Autodesk Fusion 360 part; units mm, degrees
box "BoxPrimitive1" add length 35 width 12 height 12 placed x (0, 0, -1) y (-1, 0, 0) z (0, 1, 0) at (12, 0, 0)
box "BoxPrimitive2" add length 12 width 35 height 12 placed x (0, 0, -1) y (-1, 0, 0) z (0, 1, 0) at (35, 0, 0)
box "BoxPrimitive3" add length 12 width 12 height 35 placed x (0, 0, -1) y (-1, 0, 0) z (0, 1, 0) at (12, 0, 0)
cylinder "CylinderPrimitive1" cut diameter 3 height 15 placed x (1, 0, 0) y (0, 0, -1) z (0, 1, 0) at (30, 0, -5)
cylinder "CylinderPrimitive2" cut diameter 3 height 15 placed x (1, 0, 0) y (0, 0, -1) z (0, 1, 0) at (20, 0, -5)
cylinder "CylinderPrimitive3" cut diameter 3 height 15 placed x (1, 0, 0) y (0, 0, -1) z (0, 1, 0) at (5, 0, -30)
cylinder "CylinderPrimitive4" cut diameter 3 height 15 placed x (1, 0, 0) y (0, 0, -1) z (0, 1, 0) at (5, 0, -20)
cylinder "CylinderPrimitive5" cut diameter 3 height 15 placed x (0, 0, -1) y (0, 1, 0) z (1, 0, 0) at (0, 5, -30)
cylinder "CylinderPrimitive6" cut diameter 3 height 15 placed x (0, 0, -1) y (0, 1, 0) z (1, 0, 0) at (0, 5, -20)
cylinder "CylinderPrimitive7" cut diameter 3 height -15 placed x (0, 1, 0) y (1, 0, 0) z (0, 0, -1) at (30, 5, -12)
cylinder "CylinderPrimitive8" cut diameter 3 height -15 placed x (0, 1, 0) y (1, 0, 0) z (0, 0, -1) at (20, 5, -12)
cylinder "CylinderPrimitive9" cut diameter 3 height -15 placed x (0, 0, -1) y (0, 1, 0) z (1, 0, 0) at (12, 30, -5)
cylinder "CylinderPrimitive10" cut diameter 3 height -15 placed x (0, 0, -1) y (0, 1, 0) z (1, 0, 0) at (12, 20, -5)
cylinder "CylinderPrimitive11" cut diameter 3 height -15 placed x (0, 1, 0) y (1, 0, 0) z (0, 0, -1) at (5, 30, -12)
cylinder "CylinderPrimitive12" cut diameter 3 height -15 placed x (0, 1, 0) y (1, 0, 0) z (0, 0, -1) at (5, 20, -12)
box "BoxPrimitive7" cut length 45 width 50 height 10 placed x (0, 0, -1) y (-1, 0, 0) z (0, 1, 0) at (40, 0, 0)
box "BoxPrimitive9" cut length 52 width 10 height -10 placed x (0, 1, 0) y (-1, 0, 0) z (0, 0, 1) at (10, -12, 0)
sketch "Sketch32" plane through (0, 0, -12) normal (0, 0, -1) x (-1, 0, 0)
  circle A0 centre (-5, 20) radius 1.5
  circle A1 centre (-5, 30) radius 1.5
  line L0 (-12, 12) -> (0, 12)
  line L1 (0, 12) -> (0, 35)
  line L2 (0, 35) -> (-12, 35)
  line L3 (-12, 35) -> (-12, 12)
  line L4 (-12, 35) -> (-35, 12)
  line L5 (-35, 12) -> (-12, 12)
  point P0 (-35, 12)
extrude "Extrude8" add sketch "Sketch32" against normal blind 2 contours L3 L4 L5
sketch "Sketch33" plane through (12, 0, 0) normal (1, 0, 0) x (0, 0, -1)
  line L0 (10, 12) -> (10, 35)
  line L1 (10, 35) -> (0, 35)
  line L2 (0, 35) -> (0, 12)
  line L3 (0, 12) -> (10, 12)
  circle A0 centre (5, 30) radius 1.5
  circle A1 centre (5, 20) radius 1.5
  line L4 (12, 35) -> (35, 12)
  line L5 (35, 12) -> (12, 12)
  line L6 (12, 12) -> (12, 35)
  point P0 (12, 35)
  point P1 (35, 12)
  point P2 (12, 12)
extrude "Extrude9" add sketch "Sketch33" against normal blind 2 contours L4 L5 L6
sketch "Sketch34" plane through (0, 12, 0) normal (0, 1, 0) x (-1, 0, 0)
  line L0 (-35, -10) -> (-12, -10)
  line L1 (-12, -10) -> (-12, 0)
  line L2 (-12, 0) -> (-35, 0)
  line L3 (-35, 0) -> (-35, -10)
  circle A0 centre (-30, -5) radius 1.5
  circle A1 centre (-20, -5) radius 1.5
  line L4 (-12, -35) -> (-35, -12)
  line L5 (-35, -12) -> (-12, -12)
  line L6 (-12, -12) -> (-12, -35)
  point P0 (-12, -35)
  point P1 (-35, -12)
  point P2 (-12, -12)
  point P3 (-12, -35)
extrude "Extrude10" add sketch "Sketch34" against normal blind 2 contours L4 L5 L6
cylinder "CylinderPrimitive13" cut diameter 3 height 15 placed x (1, 0, 0) y (0, 0, -1) z (0, 1, 0) at (20, 0, -20)
cylinder "CylinderPrimitive14" cut diameter 3 height -15 placed x (0, 0, -1) y (0, 1, 0) z (1, 0, 0) at (12, 20, -20)
cylinder "CylinderPrimitive15" cut diameter 3 height -15 placed x (0, 1, 0) y (1, 0, 0) z (0, 0, -1) at (20, 20, -12)
For this review, take the finished solid that the model builds, in its own axes (mm). A direction names the side the tool comes from. Round coordinates to 2 decimals unless told otherwise and drop trailing zeros. Write each loop counter-clockwise with the first axis right and the second up, starting at its lowest first coordinate (ties: lowest second). Pieces come first, ordered by that corner, then holes. Notation, with made-up numbers: (57, 51.25) - (78, 51.25) arc R9 cw to (78, 56.25) - close; hole circle Ø9 at (-16.5, 54). An arc over 180 degrees is marked (long way). Answer as a JSON object with one key per item and string values.
1. To check wall thickness, follow line 1 along Z through (x, y) = (5, 10.8); line 2 along X through (y, z) = (10.55, -5); line 3 along X through (y, z) = (20, -11). State the ranges of each line that lie inside material, in increasing order.
Response values:
{"line 1": "z = -35 to -31.5, -28.5 to -21.5, -18.5 to -10", "line 2": "x = 10 to 18.5, 21.5 to 28.5, 31.5 to 35", "line 3": "x = 0 to 3.5, 6.5 to 18.5, 21.5 to 27"}
2. We need section B-B on z = -30. Give the boundary of the cut face in (x, y).
Response values:
{"outline": "(0, 10) - (3.5, 10) - (3.5, 12) - (0, 12) - close; (6.5, 10) - (17, 10) - (17, 12) - (12, 12) - (12, 17) - (10, 17) - (10, 12) - (6.5, 12) - close"}
3. We need section C-C on x = 30. Give the boundary of the cut face in (y, z), then the cut area to 3 significant figures.
Response values:
{"outline": "(10, -17) - (12, -17) - (12, -12) - (17, -12) - (17, -10) - (12, -10) - (12, -6.5) - (10, -6.5) - close; (10, -3.5) - (12, -3.5) - (12, 0) - (10, 0) - close", "area": "38.0 mm2"}
4. For pin 1 Ø7 at (x, y) = (18.5, 26.5) entering from -Z; pin 2 Ø2.5 at (x, y) = (5, 20) entering from +Z; pin 3 Ø4 at (y, z) = (23.5, -16) entering from +X; pin 4 Ø4 at (y, z) = (18.5, -5.5) entering from -X, all flat-tipped, find the tip position at first contact; note any pin that passes through.
Response values:
{"pin 1": "stops at z = -12", "pin 2": "passes through", "pin 3": "stops at x = 12", "pin 4": "stops at x = 10"}
5. Draft analysis for pull direction X (two halves, no side actions). For faces 4 (the face through (10, 19, -18)), 5 (the face through (18.89, 11.01, -21.01)), 6 (the face through (5, 24, -12)), state which applies: +X half, -X half, draft (parallel to the pull), parting line (faces both ways), or undercut.
Response values:
{"face 4": "-X half", "face 5": "undercut", "face 6": "draft"}
6. Tool access review of faces 1 (the face through (5, 22, -10)), 2 (the face through (18.5, 18.5, -12)), 3 (the face through (28.5, 11.01, -5.07)): name each direction out of +Z, -Z, +X, -X, +Y, -Y from which nothing blocks a thin tool from reaching the whole face with its end or side.
Response values:
{"face 1": "+Z, -X, +Y, -Y", "face 2": "-Z, +X, +Y", "face 3": "+Y, -Y"}
7. We need section A-A on x = 20. Give the boundary of the cut face in (y, z).
Response values:
{"outline": "(10, -27) - (12, -27) - (12, -21.5) - (10, -21.5) - close; (10, -18.5) - (12, -18.5) - (12, -12) - (18.5, -12) - (18.5, -10) - (12, -10) - (12, -6.5) - (10, -6.5) - close; (10, -3.5) - (12, -3.5) - (12, 0) - (10, 0) - close; (21.5, -12) - (27, -12) - (27, -10) - (21.5, -10) - close"}
8. We need section D-D on y = 26.75. Give the boundary of the cut face in (x, z), then the cut area to 3 significant figures.
Response values:
{"outline": "(0, -12) - (10, -12) - (10, -20.25) - (12, -20.25) - (12, -12) - (20.25, -12) - (20.25, -10) - (12, -10) - (12, 0) - (10, 0) - (10, -10) - (0, -10) - close", "area": "77.0 mm2"}
